Could you check a few things on this model? Use its own coordinates, in mm. Round coordinates to 2 decimals unless told otherwise and drop trailing zeros. Write each loop counter-clockwise with the first axis right and the second up, starting at its lowest first coordinate (ties: lowest second). Pieces come first, ordered by that corner, then holes.
```python
from build123d import *

# Parameters (mm, degrees)
F0_R     = 2.600347
F0_R_2   = 2.5
F1_DEPTH = 3


with BuildPart() as f1:
    # F0 (on Front) → F1 (new body)
    with BuildSketch(Plane.XZ):
        with BuildLine():
            ThreePointArc((-11.107391, 30.109689), (-10.641465, 28.984844), (-11.607391, 28.243663))
            Line((-11.607391, 28.243663), (-14.897391, 28.243663))
            ThreePointArc((-14.897391, 28.243663), (-16.372391, 26.768663), (-14.897391, 25.293663))
            Line((-14.897391, 25.293663), (-11.607391, 25.293663))
            ThreePointArc((-11.607391, 25.293663), (-6.845027, 23.321027), (-4.872391, 18.558663))
            Line((-4.872391, 18.558663), (-4.872391, -27.230971))
            Line((-4.872391, -27.230971), (-4.872391, -59.108431))
            Line((-4.872391, -59.108431), (3.131261, -59.108431))
            Line((3.131261, -59.108431), (3.131261, -27.230971))
            Line((3.131261, -27.230971), (3.13126, 7.418663))
            ThreePointArc((3.13126, 7.418663), (4.715363, 15.219607), (9.216732, 21.784801))
            Line((9.216732, 21.784801), (6.36626, 23.427638))
            ThreePointArc((6.36626, 23.427638), (5.900335, 24.552482), (6.86626, 25.293663))
            Line((6.86626, 25.293663), (10.15626, 25.293663))
            ThreePointArc((10.15626, 25.293663), (11.63126, 26.768663), (10.15626, 28.243663))
            Line((10.15626, 28.243663), (6.86626, 28.243663))
            ThreePointArc((6.86626, 28.243663), (5.900335, 28.984844), (6.36626, 30.109689))
            Line((6.36626, 30.109689), (9.215484, 31.754689))
            ThreePointArc((9.215484, 31.754689), (9.755372, 33.769576), (7.740484, 34.309464))
            Line((7.740484, 34.309464), (4.89126, 32.664464))
            ThreePointArc((4.89126, 32.664464), (3.684154, 32.823382), (3.525235, 34.030489))
            Line((3.525235, 34.030489), (5.170235, 36.879713))
            ThreePointArc((5.170235, 36.879713), (4.630348, 38.8946), (2.61546, 38.354713))
            Line((2.61546, 38.354713), (0.97046, 35.505489))
            ThreePointArc((0.97046, 35.505489), (-0.154384, 35.039563), (-0.895565, 36.005489))
            Line((-0.895565, 36.005489), (-0.895565, 39.295489))
            ThreePointArc((-0.895565, 39.295489), (-2.370565, 40.770489), (-3.845565, 39.295489))
            Line((-3.845565, 39.295489), (-3.845565, 36.005489))
            ThreePointArc((-3.845565, 36.005489), (-4.586746, 35.039563), (-5.711591, 35.505489))
            Line((-5.711591, 35.505489), (-7.356591, 38.354713))
            ThreePointArc((-7.356591, 38.354713), (-9.371478, 38.8946), (-9.911366, 36.879713))
            Line((-9.911366, 36.879713), (-8.266366, 34.030489))
            ThreePointArc((-8.266366, 34.030489), (-8.425284, 32.823382), (-9.632391, 32.664464))
            Line((-9.632391, 32.664464), (-12.481615, 34.309464))
            ThreePointArc((-12.481615, 34.309464), (-14.496502, 33.769576), (-13.956615, 31.754689))
            Line((-13.956615, 31.754689), (-11.107391, 30.109689))
        make_face()
        with Locations((-0.91964, -52.217755)):
            Circle(F0_R, mode=Mode.SUBTRACT)
        with Locations((-0.892788, -28.898051)):
            Circle(F0_R, mode=Mode.SUBTRACT)
        with Locations((-2.372391, 26.768663)):
            Circle(F0_R_2, mode=Mode.SUBTRACT)
        with Locations((-0.91964, -7.323526)):
            Circle(F0_R, mode=Mode.SUBTRACT)
    extrude(amount=F1_DEPTH)


solid = f1.part
```
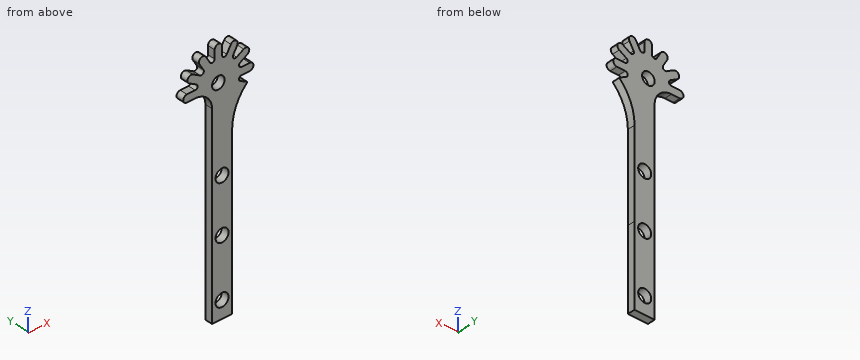
Q1. If I drill on L1, parallel to Z at x = 8, y = -2.1; L2, parallel to Z at x = 1, y = -2.75; L3, parallel to Z at x = 6.25, y = -0.4, over which ranges is the centre line in solid material (lowest first)?
Q2. I'm going to push flat-ended pins straight in: pin 1 Ø1.5 at (x, y) = (8.5, -2) entering from +Z; pin 2 Ø0.9 at (y, z) = (-1.5, -36) entering from +X; pin 3 Ø1.5 at (x, y) = (-12.5, -1) entering from -Z; pin 4 Ø10 at (x, z) = (-7.5, -45.5) entering from +Y. Where does each tip first touch, or does it pass through?
Q3. Imagine slicing it at B-B, the plane y = -2. Count the separate pieces of the cut face and the enclosed holes in it, then the cut area to 3 significant figures.
Q4. Imagine slicing it at A-A, the plane z = -22.5. Write out the boundary of the cut face in (x, y), then the cut area to 3 significant figures.
Results found:
1. L1: z = 20.5 to 22.49, 25.29 to 28.24, 31.05 to 34.43
1. L2: z = -59.11 to -53.97, -50.46 to -30.68, -27.12 to -9.08, -5.57 to 35.56
1. L3: z = 18.14 to 23.51, 25.08 to 28.46, 30.03 to 33.45
2. pin 1: stops at z = 34.51
2. pin 2: stops at x = 3.13
2. pin 3: stops at z = 25.29
2. pin 4: stops at y = 0
3. separate pieces: 1
3. enclosed holes: 4
3. area: 891 mm2
4. outline: (-4.87, -3) - (3.13, -3) - (3.13, 0) - (-4.87, 0) - close
4. area: 24.0 mm2
